Can you work these out from the drawing? Everything is in mm from the part's minimum corner. Coordinates: 2 decimals unless noted, no trailing zeros. Order: outer loops, then holes, each group sorted by start corner. A loop starts at its lowest first (then second) coordinate and runs counter-clockwise, first axis right, second up. Notation, with made-up numbers: (-19.75, -26) -> (11.25, -26) arc R26 cw to (11.25, 0) -> close; hole circle Ø2 at (76, -1.75). An arc over 180 degrees is marked (long way). Use a Markdown table: item, result. Add a question column.
1) If I drill on L1, parallel to X at y = 6, z = 17; L2, parallel to Z at x = 14.5, y = 6; L3, parallel to X at y = 4, z = 43, over which ranges is the centre line in solid material (lowest first)? Write a range as [from, to].
2) If we section it at B-B (z = 43.5): Write out the boundary of the cut face in (x, y), plus the area to 3 significant figures.
3) If we section it at A-A (x = 52): Write out the boundary of the cut face in (y, z).
4) If we section it at C-C (z = 69): Write out the boundary of the cut face in (x, y), plus the area to 3 significant figures.
5) Will these pins go through, and if not, where does the flat tip stop? pin 1 Ø1.1 at (x, y) = (7, 2) entering from +Z; pin 2 Ø3 at (x, y) = (7, 3) entering from -Z; pin 3 Ø1.5 at (y, z) = (4, 38.5) entering from -X.
6) Thinking about a two-plate mould opening in Z: for the marked faces 1 and 2, which applies, +Z half, -Z half, draft (parallel to the pull), parting line (faces both ways), or undercut?
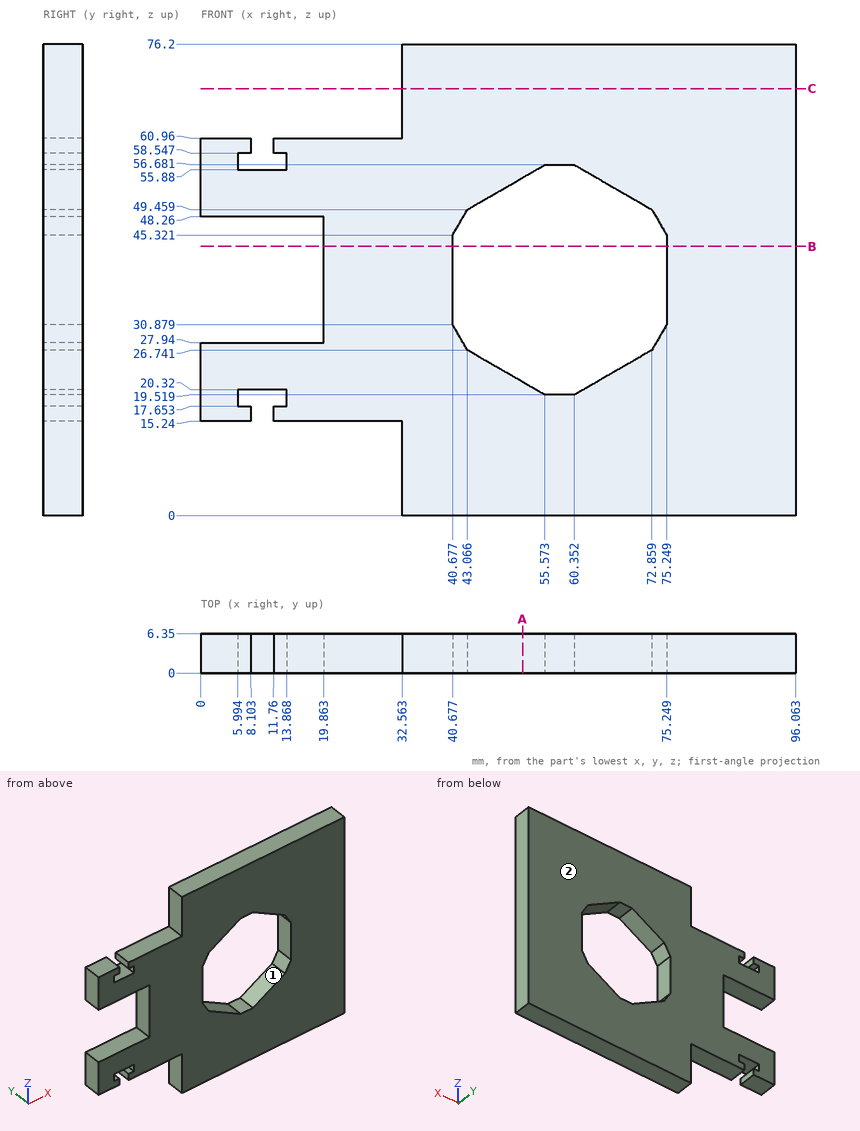
Answer sheet:
| question | item | result |
|---|---|---|
| 1 | L1 | [0, 8.1], [11.76, 96.06] |
| 1 | L2 | [15.24, 27.94], [48.26, 60.96] |
| 1 | L3 | [19.86, 40.68], [75.25, 96.06] |
| 2 | outline | (19.86, 0) -> (40.68, 0) -> (40.68, 6.35) -> (19.86, 6.35) -> close; (75.25, 0) -> (96.06, 0) -> (96.06, 6.35) -> (75.25, 6.35) -> close |
| 2 | area | 264 mm2 |
| 3 | outline | (0, 0) -> (6.35, 0) -> (6.35, 21.58) -> (0, 21.58) -> close; (0, 54.62) -> (6.35, 54.62) -> (6.35, 76.2) -> (0, 76.2) -> close |
| 4 | outline | (32.56, 0) -> (96.06, 0) -> (96.06, 6.35) -> (32.56, 6.35) -> close |
| 4 | area | 403 mm2 |
| 5 | pin 1 | z = 60.96 |
| 5 | pin 2 | z = 15.24 |
| 5 | pin 3 | x = 19.86 |
| 6 | face 1 | undercut |
| 6 | face 2 | draft |
